Input: part model. Units: mm. Frame: model coordinates. Face numbers are marked on the shaded views. A direction names the side the tool comes from. Coordinates: 2 decimals unless noted, no trailing zeros. Write each loop counter-clockwise with the first axis right and the second up, starting at its lowest first coordinate (ties: lowest second). Pieces come first, ordered by that corner, then holes.
1) Section query A-A (x = 37.5). Output: boundary loops of the cut face in (y, z), then the cut area to 3 significant figures.
2) Section query C-C (z = 56.5). Output: boundary loops of the cut face in (x, y).
3) Draft query along Y for the marked faces 1, 2 and 3. Return one class per face: pulls with the +Y half, pulls with the -Y half, needs draft (parallel to the pull), parting line crosses it, or undercut.
4) Set-up query: the marked faces 4 and 5. Return all of +Z, -Z, +X, -X, +Y, -Y with unobstructed straight access to the full face (end or side cutting, diameter ignored); none if empty.
5) Pin query (flat end, axial travel): pin 1 Ø22.5 at (x, z) = (20, 112) entering from +Y. Return the tip coordinate at first contact, or that it passes through.
6) Line query: L1, parallel to Y at x = 39.6, z = 163; L2, parallel to X at y = 20, z = 124.5. Output: solid intervals per line, ascending.
7) Section query D-D (z = 163). Output: boundary loops of the cut face in (x, y), then the cut area to 3 significant figures.
from build123d import *

# Parameters (mm, degrees)
SKETCH_1_W          = 40
SKETCH_1_H          = 40
SKETCH_1_W_2        = 38
SKETCH_1_H_2        = 38
EXTRUDE_1_DEPTH     = 170
SKETCH_2_R          = 2.1
CUT_EXTRUDE_1_DEPTH = 180.164728672
SKETCH_12_R         = 1.6
CUT_EXTRUDE_2_DEPTH = 180.164728672
SKETCH_13_R         = 1.6
CUT_EXTRUDE_3_DEPTH = 180.164728672
SKETCH_14_R         = 12.5
CUT_EXTRUDE_4_DEPTH = 180.164728672


with BuildPart() as part:
    # 草图1 → 凸台-拉伸1 (new body)
    with BuildSketch(Plane.XY):
        with Locations((20, 20)):
            Rectangle(SKETCH_1_W, SKETCH_1_H)
        with Locations((20, 20)):
            Rectangle(SKETCH_1_W_2, SKETCH_1_H_2, mode=Mode.SUBTRACT)
    extrude(amount=EXTRUDE_1_DEPTH)

    # 草图2 → 切除-拉伸1 (cut, through all)
    with BuildSketch(Plane.XZ):
        with Locations(Location((8, 6, 0), (0, 0, 270))):
            Circle(SKETCH_2_R)
        with Locations(Location((32, 22, 0), (0, 0, 270))):
            Circle(SKETCH_2_R)
        with Locations(Location((8, 22, 0), (0, 0, 270))):
            Circle(SKETCH_2_R)
        with Locations(Location((32, 6, 0), (0, 0, 270))):
            Circle(SKETCH_2_R)
    extrude(amount=-CUT_EXTRUDE_1_DEPTH, mode=Mode.SUBTRACT)

    # 草图12 → 切除-拉伸2 (cut, through all)
    with BuildSketch(Plane.ZY):
        with Locations((112.92, 7)):
            Circle(SKETCH_12_R)
        with Locations((94.92, 7)):
            Circle(SKETCH_12_R)
        with Locations((76.92, 7)):
            Circle(SKETCH_12_R)
        with Locations((94.92, 23)):
            Circle(SKETCH_12_R)
        with Locations((76.92, 23)):
            Circle(SKETCH_12_R)
        with Locations((112.92, 23)):
            Circle(SKETCH_12_R)
    extrude(amount=-CUT_EXTRUDE_2_DEPTH, mode=Mode.SUBTRACT)

    # 草图13 → 切除-拉伸3 (cut, through all)
    with BuildSketch(Plane.ZY):
        with Locations((163, 29.343081894)):
            Circle(SKETCH_13_R)
        with Locations((163, 10)):
            Circle(SKETCH_13_R)
        with Locations((148.01439139, 29.999994822)):
            Circle(SKETCH_13_R)
        with Locations((148, 10)):
            Circle(SKETCH_13_R)
    extrude(amount=-CUT_EXTRUDE_3_DEPTH, mode=Mode.SUBTRACT)

    # 草图14 → 切除-拉伸4 (cut, through all)
    with BuildSketch(Plane.XZ):
        with Locations(Location((20, 42, 0), (0, 0, 270))):
            Circle(SKETCH_14_R)
        with Locations(Location((20, 77, 0), (0, 0, 270))):
            Circle(SKETCH_14_R)
        with Locations(Location((20, 112, 0), (0, 0, 270))):
            Circle(SKETCH_14_R)
        with Locations(Location((20, 147, 0), (0, 0, 270))):
            Circle(SKETCH_14_R)
    extrude(amount=-CUT_EXTRUDE_4_DEPTH, mode=Mode.SUBTRACT)


solid = part.part
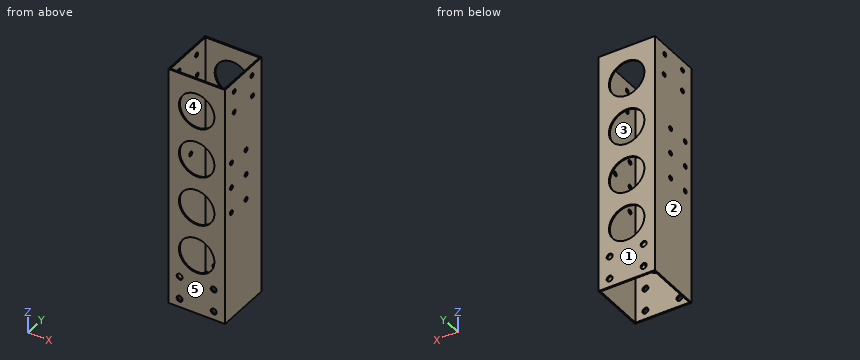
Answer:
1. outline: (0, 0) - (1, 0) - (1, 170) - (0, 170) - close; (39, 0) - (40, 0) - (40, 170) - (39, 170) - close
1. area: 340 mm2
2. outline: (0, 0) - (40, 0) - (40, 40) - (0, 40) - close; hole (1, 1) - (39, 1) - (39, 39) - (1, 39) - close
3. face 1: pulls with the +Y half
3. face 2: needs draft
3. face 3: undercut
4. face 4: +Z, -Z
4. face 5: +Z, -Z, +X, -X, -Y
5. pin 1: passes through
6. L1: y = 0 to 8.4, 11.6 to 27.74, 30.94 to 40
6. L2: x = 0 to 1, 39 to 40
7. outline: (0, 0) - (40, 0) - (40, 8.4) - (39, 8.4) - (39, 1) - (1, 1) - (1, 8.4) - (0, 8.4) - close; (0, 11.6) - (1, 11.6) - (1, 27.74) - (0, 27.74) - close; (0, 30.94) - (1, 30.94) - (1, 39) - (39, 39) - (39, 30.94) - (40, 30.94) - (40, 40) - (0, 40) - close; (39, 11.6) - (40, 11.6) - (40, 27.74) - (39, 27.74) - close
7. area: 143 mm2
